from build123d import *

# Parameters (mm, degrees)
F1_DEPTH = 304.8
F3_DEPTH = 25.4
F5_DEPTH = 25.4
F7_DEPTH = 25.4
F9_DEPTH = 25.4


with BuildPart() as f1:
    # F0 (on Front) → F1 (new body)
    with BuildSketch(Plane.XZ):
        Polygon((-2.54, 0), (0, 0), (0, 38.1), (-2.54, 38.1), (-2.54, 20.955), (-25.4, 20.955), (-25.4, 19.05), (-2.54, 19.05), (-2.54, 15.24), (-5.08, 15.24), (-5.08, 12.446), (-3.81, 12.446), (-3.81, 13.97), (-2.54, 13.97), (-2.54, 7.62), (-3.81, 7.62), (-3.81, 9.144), (-5.08, 9.144), (-5.08, 6.35), (-2.54, 6.35), align=None)
    extrude(amount=F1_DEPTH)

    # F2 (on face) → F3 (cut)
    with BuildSketch(Plane.YZ):
        Polygon((-266.7, 0), (-304.8, 38.1), (-304.8, 0), align=None)
        Polygon((0, 0), (0, 38.1), (-38.1, 0), align=None)
    extrude(amount=-F3_DEPTH, mode=Mode.SUBTRACT)

    # F4 (on face) → F5 (cut)
    with BuildSketch(Plane.XY.offset(20.955)):
        Polygon((-25.4, -37.465), (-2.54, -17.145), (-25.4, -17.145), align=None)
        Polygon((-25.4, -287.655), (-2.54, -287.655), (-25.4, -267.335), align=None)
    extrude(amount=-F5_DEPTH, mode=Mode.SUBTRACT)

    # F6 (on face) → F7 (cut)
    with BuildSketch(Plane.XY.offset(20.955)):
        with BuildLine():
            Line((-13.97, -39.794183), (-20.32, -39.794183))
            ThreePointArc((-20.32, -39.794183), (-23.1775, -42.651683), (-20.32, -45.509183))
            Line((-20.32, -45.509183), (-13.97, -45.509183))
            ThreePointArc((-13.97, -45.509183), (-11.1125, -42.651683), (-13.97, -39.794183))
        make_face()
        with BuildLine():
            Line((-20.32, -265.005817), (-13.97, -265.005817))
            ThreePointArc((-13.97, -265.005817), (-11.1125, -262.148317), (-13.97, -259.290817))
            Line((-13.97, -259.290817), (-20.32, -259.290817))
            ThreePointArc((-20.32, -259.290817), (-23.1775, -262.148317), (-20.32, -265.005817))
        make_face()
    extrude(amount=-F7_DEPTH, mode=Mode.SUBTRACT)

    # F8 (on face) → F9 (cut)
    with BuildSketch(Plane.YZ):
        Polygon((-15.24, 22.86), (0, 38.1), (-15.24, 38.1), align=None)
    extrude(amount=-F9_DEPTH, mode=Mode.SUBTRACT)


solid = f1.part
Design review of the part built by this model. Coordinates are the model's own, in mm. A direction names the side the tool comes from. Coordinates: 2 decimals unless noted, no trailing zeros. Write each loop counter-clockwise with the first axis right and the second up, starting at its lowest first coordinate (ties: lowest second). Pieces come first, ordered by that corner, then holes. Notation, with made-up numbers: (-39, -7.5) - (1, -7.5) arc R15 cw to (1, 11.5) - close; hole circle Ø4 at (37.5, -4.5). An arc over 180 degrees is marked (long way). One line per item, written item: value.
1) Mouldability with a two-part tool opening along X and no side actions: class faces 1 (the face through (-2.54, -151, 11)), 2 (the face through (0, -158, 19)), 3 (the face through (-13.81, -277.637, 20.016)) as +X half, -X half, draft (parallel to the pull), parting line (faces both ways), or undercut.
Answer sheet:
face 1: undercut
face 2: +X half
face 3: -X half
2) To check wall thickness, follow probe 1 along Z at (x, y) = (-3, -88) (3 decimals); probe 2 along Z at (x, y) = (-23, -171) (3 decimals); probe 3 along X at (y, z) = (-41.5, 20). State the ranges of each line that lie inside material, in increasing order.
Answer sheet:
probe 1: z = 6.35 to 7.62, 13.97 to 15.24, 19.05 to 20.955
probe 2: z = 19.05 to 20.955
probe 3: x = -25.4 to -22.94, -11.35 to 0
3) Add section A-A (x = -16.5). State the section outline as (y, z) points (3 decimals), plus the area to 3 significant figures.
Answer sheet:
outline: (-275.246, 19.05) - (-265.006, 19.05) - (-265.006, 20.955) - (-275.246, 20.955) - close; (-259.291, 19.05) - (-45.509, 19.05) - (-45.509, 20.955) - (-259.291, 20.955) - close; (-39.794, 19.05) - (-29.554, 19.05) - (-29.554, 20.955) - (-39.794, 20.955) - close
area: 446 mm2
4) Add section B-B (y = -239). State the section outline as (x, z) points (3 decimals).
Answer sheet:
outline: (-25.4, 19.05) - (-2.54, 19.05) - (-2.54, 15.24) - (-5.08, 15.24) - (-5.08, 12.446) - (-3.81, 12.446) - (-3.81, 13.97) - (-2.54, 13.97) - (-2.54, 7.62) - (-3.81, 7.62) - (-3.81, 9.144) - (-5.08, 9.144) - (-5.08, 6.35) - (-2.54, 6.35) - (-2.54, 0) - (0, 0) - (0, 38.1) - (-2.54, 38.1) - (-2.54, 20.955) - (-25.4, 20.955) - close
5) For faces 4 (the face through (-1.4, -285.5, 18.8)), 5 (the face through (-2.54, -158, 30)), 6 (the face through (-2.54, -151, 3)), list the 3-axis set-ups (+Z, -Z, +X, -X, +Y, -Y) from which the entire face can be reached by the end or side of a thin tool; tool diameter is ignored.
Answer sheet:
face 4: -Z, +X, -X, -Y
face 5: +Z, -X, +Y, -Y
face 6: -Z, -X, +Y, -Y
6) Add section C-C (z = 35.5). State the section outline as (x, y) points, plus the area to 3 significant figures.
Answer sheet:
outline: (-2.54, -302.2) - (0, -302.2) - (0, -15.24) - (-2.54, -15.24) - close
area: 729 mm2
7) Insertion check: pin 1 (1.2 mm diameter, centred on y = -191.5, z = 13, fed in from +X); pin 2 (10 mm diameter, centred on x = -13.5, y = -245, fed in from -Z); pin 3 (1 mm diameter, centred on y = -75, z = 24.5, fed in from -X); pin 4 (0.8 mm diameter, centred on x = -4, y = -122, fed in from +Z) (3 decimals). Each pin has a flat end and moves straight along its axis. Give the tip position at first contact, or say it passes through.
Answer sheet:
pin 1: stops at x = 0
pin 2: stops at z = 19.05
pin 3: stops at x = -2.54
pin 4: stops at z = 20.955
